The listing builds one solid part. Answer for the finished solid, in the listing's coordinates (mm). Face numbers are marked on the shaded views. A direction names the side the tool comes from. Round coordinates to 2 decimals unless told otherwise and drop trailing zeros. Loops run counter-clockwise (first coordinate to the right, second up) from the corner with the lowest first, then second, coordinate; pieces in that order, holes last. Notation, with made-up numbers: (61, -33) -> (117, -33) arc R4 cw to (117, -27) -> close; hole circle Ø11 at (54.25, 57). An arc over 180 degrees is marked (long way). Use a Markdown table: item, result. Add a question column.
Q1. Section D-D on z = -3.5 is taken. Give the vertices of the cut face in (x, y).
Q2. Consider line 1 (Z direction, x = -9.5, y = -25); line 2 (Z direction, x = 35.5, y = 17.5); line 3 (X direction, y = 14, z = 46.5). Determine where each line is inside the solid, lowest interval first.
Q3. Which of the six approach directions +Z, -Z, +X, -X, +Y, -Y give full straight-line access (tool end or side, diameter ignored) to the marked faces 1, 2 and 3?
Q4. For a pull along X with two mould halves and no side action, classify the marked faces 4, 5, 6 and 7 as released by +X, released by -X, zero draft, split by the parting line, or undercut.
Q5. Section A-A on x = 0 is taken. Give the vertices of the cut face in (y, z), then the cut area to 3 significant figures.
Q6. Given pin 1 Ø12 at (x, y) = (2.5, 31.5) entering from -Z; pin 2 Ø20.5 at (x, y) = (26.5, -1) entering from +Z; pin 3 Ø10 at (x, y) = (-13.5, 31) entering from +Z, each flat-ended and moving along its own axis, determine where each tip first touches the part or whether it passes through.
Q7. Section B-B on y = 8 is taken. Give the vertices of the cut face in (x, z).
Q8. Section C-C on z = 44 is taken. Give the vertices of the cut face in (x, y) (3 decimals).
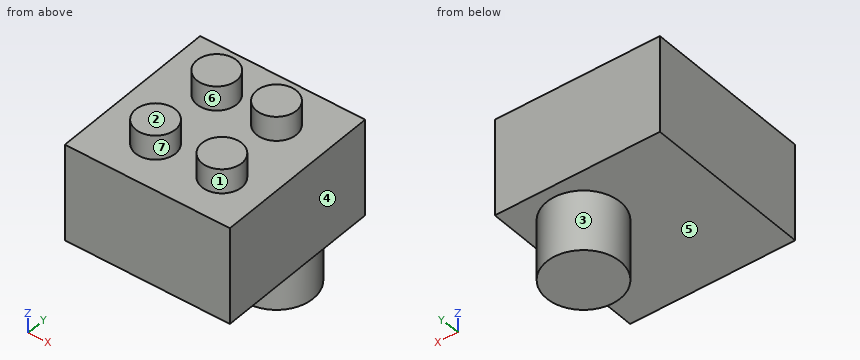
from build123d import *

# Parameters (mm, degrees)
F0_W     = 68.447597
F0_H     = 70.646504
F1_DEPTH = 40.386
F2_R     = 15.24
F3_DEPTH = 65.532
F4_R     = 8.255
F5_DEPTH = 10.16


with BuildPart() as f1:
    # F0 (on Top) → F1 (new body)
    with BuildSketch(Plane.XY):
        with Locations((11.513501, 5.437753)):
            Rectangle(F0_W, F0_H)
    extrude(amount=F1_DEPTH)

    # F2 (on face) → F3 (join)
    with BuildSketch(Plane.XY.offset(40.386)):
        with Locations((24.792334, 20.836459)):
            Circle(F2_R)
    extrude(amount=-F3_DEPTH)

    # F4 (on face) → F5 (join)
    with BuildSketch(Plane.XY.offset(40.386)):
        with Locations((0, 20.836459)):
            Circle(F4_R)
        with Locations((0, -11.11847)):
            Circle(F4_R)
        with Locations((24.792334, 20.836459)):
            Circle(F4_R)
        with Locations((27.5301, -11.11847)):
            Circle(F4_R)
    extrude(amount=F5_DEPTH)


solid = f1.part
Checked values:
| question | item | result |
|---|---|---|
| 1 | outline | circle Ø30.48 at (24.79, 20.84) |
| 2 | line 1 | z = 0 to 40.39 |
| 2 | line 2 | z = -25.15 to 40.39 |
| 2 | line 3 | x = -4.63 to 4.63, 20.17 to 29.42 |
| 3 | face 1 | +Z |
| 3 | face 2 | +Z, +X, -X, +Y, -Y |
| 3 | face 3 | -Z |
| 4 | face 4 | released by +X |
| 4 | face 5 | zero draft |
| 4 | face 6 | undercut |
| 4 | face 7 | undercut |
| 5 | outline | (-29.89, 0) -> (40.76, 0) -> (40.76, 40.39) -> (29.09, 40.39) -> (29.09, 50.55) -> (12.58, 50.55) -> (12.58, 40.39) -> (-2.86, 40.39) -> (-2.86, 50.55) -> (-19.37, 50.55) -> (-19.37, 40.39) -> (-29.89, 40.39) -> close |
| 5 | area | 3,190 mm2 |
| 6 | pin 1 | stops at z = 0 |
| 6 | pin 2 | stops at z = 50.55 |
| 6 | pin 3 | stops at z = 40.39 |
| 7 | outline | (-22.71, 0) -> (16.58, 0) -> (16.58, -25.15) -> (33.01, -25.15) -> (33.01, 0) -> (45.74, 0) -> (45.74, 40.39) -> (-22.71, 40.39) -> close |
| 8 | outline | circle Ø16.51 at (0, -11.118); circle Ø16.51 at (0, 20.836); circle Ø16.51 at (24.792, 20.836); circle Ø16.51 at (27.53, -11.118) |
